```python
from build123d import *

# Parameters (mm, degrees)
F1_DEPTH = 10
F2_R     = 5
F4_DEPTH = 10.001
F5_R     = 5
F7_D     = 4.2
F7_DEPTH = 10.001
F9_D     = 4.3
F9_DEPTH = 15
F9_TIP   = 1.2918503309


with BuildPart() as f1:
    # F0 (on Front) → F1 (new body)
    with BuildSketch(Plane.XZ):
        Polygon((0, 70), (0, 0), (120, 0), (120, 22), align=None)
    extrude(amount=F1_DEPTH)

    # F2
    f2_edges = [f1.edges().sort_by_distance(p)[0] for p in [
        (120, -5, 22),
    ]]
    fillet(f2_edges, radius=F2_R)

    # F3 (on Front) → F4 (cut, through all)
    with BuildSketch(Plane.XZ):
        Polygon((10, 55.2296703857), (10, 10), (110, 10), (110, 15.2296703857), align=None)
    extrude(amount=F4_DEPTH, mode=Mode.SUBTRACT)

    # F5
    f5_edges = [f1.edges().sort_by_distance(p)[0] for p in [
        (10, -5, 10),
    ]]
    fillet(f5_edges, radius=F5_R)

    # F7 (through all, one way)
    with BuildSketch(Plane.XY.offset(10)):
        with Locations((80, -5), (105, -5)):
            Circle(F7_D / 2)
    extrude(amount=-F7_DEPTH, mode=Mode.SUBTRACT)

    # F9
    with Locations(Plane(origin=(0, 0, 0), x_dir=(0, 1, 0), z_dir=(-1, 0, 0))):
        with Locations((-5, -38), (-5, -18)):
            Hole(F9_D / 2, depth=F9_DEPTH)
            with Locations((0, 0, -(F9_DEPTH + F9_TIP / 2))):  # 118° drill point
                Cone(0, F9_D / 2, F9_TIP, mode=Mode.SUBTRACT)


solid = f1.part
```
Geometry check sheet. Reference: the model listing, model coordinates, mm. A direction names the side the tool comes from. Give positions to 0.01 mm unless a question says otherwise; leave off trailing zeros. Order: outer loops, then holes, each group sorted by start corner. A loop starts at its lowest first (then second) coordinate and runs counter-clockwise, first axis right, second up. Notation, with made-up numbers: (-19, 33.25) - (-12, 33.25) arc R24 cw to (-12, 62.25) - close; hole circle Ø3 at (-11, 57.5). An arc over 180 degrees is marked (long way). Answer in a Markdown table with one row per item. Add a question column.
Q1. Cross-section at A-A, the plane y = -5. Enter the section's corners in (x, z).
Q2. Cross-section at C-C, the plane z = 38. Enter the section's corners in (x, y).
Q3. Gauge pin test, flat ends, axial feed: pin 1 (3.5 mm diameter, centred on x = 80, y = -5, fed in from -Z); pin 2 (6 mm diameter, centred on y = -2.5, z = 51.5, fed in from +X); pin 3 (2.5 mm diameter, centred on x = 105, y = -5, fed in from +Z). Record the tip position at first contact, or that the pin passes through.
Q4. Material ranges on probe 1 along Y at (x, z) = (105, 4.25); probe 2 along X at (y, z) = (-1, 14.5); probe 3 along Z at (x, y) = (7.5, -6), recorded low to high. Write a range as from..to.
Q5. Tool access check on faces 1 (the flat face through (60, 0, 38)), 2 (the cylindrical face through (102.9, -4.91, 5.07)), 3 (the flat face through (10, -5, 35)), 4 (the cylindrical face through (5.07, -4.53, 20.1)). Record the directions out of +Z, -Z, +X, -X, +Y, -Y that give a thin tool (end or side, any length) a straight path to the whole face; none if there is none.
Q6. Cross-section at B-B, the plane x = 105. Enter the section's corners in (y, z), then the cut area to 3 significant figures.
Q7. Mould release check, pull along Y, two halves, no side actions. Record for faces 5 (the cylindrical face through (77.9, -4.91, 5.07)), 6 (the flat face through (62, -5, 10)), 7 (the cylindrical face through (5.07, -4.72, 35.87)), 8 (the flat face through (60, -10, 38)): pulls with the +Y half, pulls with the -Y half, needs draft (parallel to the pull), parting line crosses it, or undercut.
Check values:
| question | item | result |
|---|---|---|
| 1 | outline | (0, 0) - (77.9, 0) - (77.9, 10) - (15, 10) arc R5 cw to (10, 15) - (10, 15.85) - (0, 15.85) - close; (0, 20.15) - (10, 20.15) - (10, 35.85) - (0, 35.85) - close; (0, 40.15) - (10, 40.15) - (10, 55.23) - (110, 15.23) - (110, 10) - (107.1, 10) - (107.1, 0) - (120, 0) - (120, 18.61) arc R5 ccw to (116.86, 23.26) - (0, 70) - close; (82.1, 0) - (102.9, 0) - (102.9, 10) - (82.1, 10) - close |
| 2 | outline | (0, -10) - (10, -10) - (10, -7.15) - (0, -7.15) - close; (0, -2.85) - (10, -2.85) - (10, 0) - (0, 0) - close; (53.07, -10) - (80, -10) - (80, 0) - (53.07, 0) - close |
| 3 | pin 1 | stops at z = 26.53 |
| 3 | pin 2 | stops at x = 53.75 |
| 3 | pin 3 | stops at z = 28.5 |
| 4 | probe 1 | y = -10..-7.1, -2.9..0 |
| 4 | probe 2 | x = 0..10.03, 110..120 |
| 4 | probe 3 | z = 0..16.1, 19.9..36.1, 39.9..67 |
| 5 | face 1 | +Z, -Z, +X, -X, +Y |
| 5 | face 2 | -Z |
| 5 | face 3 | +Y, -Y |
| 5 | face 4 | -X |
| 6 | outline | (-10, 0) - (-7.1, 0) - (-7.1, 10) - (-10, 10) - close; (-10, 17.23) - (0, 17.23) - (0, 28) - (-10, 28) - close; (-2.9, 0) - (0, 0) - (0, 10) - (-2.9, 10) - close |
| 6 | area | 166 mm^2 |
| 7 | face 5 | undercut |
| 7 | face 6 | needs draft |
| 7 | face 7 | undercut |
| 7 | face 8 | pulls with the -Y half |
